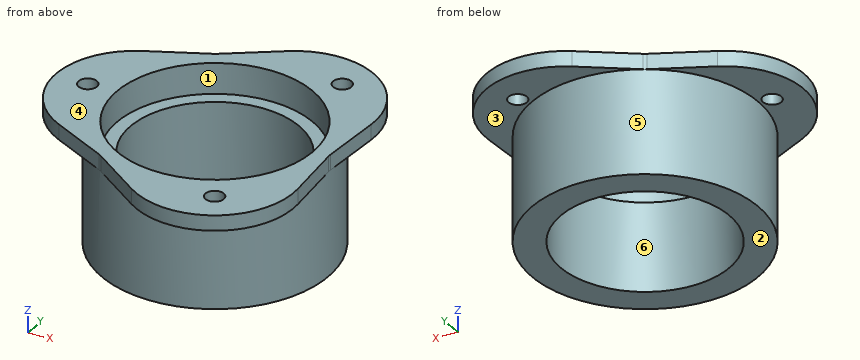
Autodesk Inventor part; units mm, degrees
ref_plane "XZ Plane" through (0, 0, 0) normal (0, 1, 0) x (-1, 0, 0)
ref_plane "XY Plane" through (0, 0, 0) normal (0, 0, 1) x (1, 0, 0)
sketch "Sketch1" plane through (0, 0, 0) normal (0, 0, 1) x (1, 0, 0)
  circle A0 centre (0, 0) radius 27.575
  circle A1 centre (0, 0) radius 51.5
  dimension "d0" = 55.15
  dimension "d1" = 103
extrude "Extrusion1" add sketch "Sketch1" along normal blind 39
sketch "Sketch2" plane through (0, 0, 0) normal (1, 0, 0) x (0, 1, 0)
  line L0 (51.5, 39) -> (-51.5, 39)
  line L1 (51.5, 0) -> (-51.5, 0)
  line L2 (42.7787, 29) -> (-54.5799, 29) construction
  line L3 (-27.575, 39) -> (27.575, 39)
  line L4 (-27.575, 39) -> (27.575, 39)
  line L5 (-27.575, 0) -> (27.575, 0)
  line L6 (51.5, 0) -> (27.575, 0)
  line L7 (27.575, 0) -> (27.575, 39)
  line L8 (27.575, 39) -> (51.5, 39)
  line L9 (-51.5, 39) -> (-27.575, 39)
  line L10 (-27.575, 39) -> (-27.575, 0)
  line L11 (-27.575, 0) -> (-51.5, 0)
  line L12 (27.575, 39) -> (32, 39)
  line L13 (32, 39) -> (32, 29)
  line L14 (32, 29) -> (27.575, 29)
  line L15 (27.575, 29) -> (27.575, 39)
  line L16 (0, -7.8) -> (0, 46.8)
  line L17 (51.5, 39) -> (51.5, 0)
  line L18 (-51.5, 0) -> (-51.5, 39)
  point P0 (0, 0)
  dimension "d4" = 10
  dimension "d5" = 32
revolve "Revolution1" cut sketch "Sketch2" angle 360 about axis through (0, 0, -10) along (0, 0, 1) contours L13 L14 L7 L0
sketch "Sketch3" plane through (0, 0, 0) normal (1, 0, 0) x (0, 1, 0)
  line L0 (51.5, 39) -> (51.5, 0)
  line L1 (51.5, 0) -> (27.575, 0)
  line L2 (27.575, 0) -> (27.575, 29)
  line L3 (27.575, 29) -> (32, 29)
  line L4 (32, 29) -> (32, 39)
  line L5 (32, 39) -> (51.5, 39)
  line L6 (-51.5, 0) -> (-51.5, 39)
  line L7 (-51.5, 39) -> (-32, 39)
  line L8 (-32, 39) -> (-32, 29)
  line L9 (-32, 29) -> (-27.575, 29)
  line L10 (-27.575, 29) -> (-27.575, 0)
  line L11 (-27.575, 0) -> (-51.5, 0)
  line L12 (-51.5, 0) -> (-51.5, 39)
  line L13 (-32, 39) -> (-32, 29)
  line L14 (-32, 34) -> (-51.5, 34)
  line L15 (-37, 34) -> (-37, 0)
  line L16 (51.5, 0) -> (-51.5, 0)
  line L17 (0, -7.8) -> (0, 46.8)
  point P0 (0, 0)
  point P1 (-51.5, 34)
  dimension "d7" = 5
  dimension "d11" = 5
revolve "Revolution2" cut sketch "Sketch3" angle 360 about axis through (0, 0, -10) along (0, 0, 1) contours L11 L6 L14 L15
sketch "Sketch4" plane through (0, 0, 39) normal (0, 0, 1) x (1, 0, 0)
  circle A0 centre (0, 0) radius 32
  circle A1 centre (0, 0) radius 51.5
  circle A2 centre (0, 0) radius 32
  line L0 (0, 0) -> (-55.0177, 0) construction
  line L1 (0, 0) -> (34.9883, -60.6016) construction
  line L2 (0, 0) -> (42.9469, 74.3862) construction
  circle A3 centre (-25.75, 0) radius 25.75 construction
  circle A4 centre (12.875, -22.3002) radius 25.75 construction
  circle A5 centre (0, 0) radius 51.5
  circle A6 centre (12.875, 22.3002) radius 25.75 construction
  line L3 (0, 0) -> (-33.8932, -58.7048) construction
  line L4 (0, 0) -> (-35.029, 60.6721) construction
  line L5 (0, 0) -> (41.9391, 0) construction
  circle A7 centre (-22.125, -38.3216) radius 7.25 construction
  circle A8 centre (-22.125, 38.3216) radius 7.25 construction
  circle A9 centre (44.25, 0) radius 7.25 construction
  line L6 (38.5484, -20.3161) -> (37.0216, -0.5586)
  line L7 (38.5484, 20.3161) -> (37.0216, 0.5586)
  line L8 (-1.68, -43.542) -> (-18.027, -32.3409)
  line L9 (-36.8684, -23.2259) -> (-18.9946, -31.7823)
  line L10 (-36.8684, 23.2259) -> (-18.9946, 31.7823)
  line L11 (-18.027, 32.3409) -> (-1.68, 43.542)
  arc A10 (-1.68, -43.542) -> (38.5484, -20.3161) centre (12.875, -22.3002) ccw
  arc A11 (37.0216, 0.5586) -> (37.0216, -0.5586) centre (44.25, 0) ccw
  arc A12 (36.3356, 11.6859) -> (-1.68, 43.542) centre (12.875, 22.3002) ccw
  arc A13 (-18.9946, 31.7823) -> (-18.027, 32.3409) centre (-22.125, 38.3216) ccw
  arc A14 (-18.027, -32.3409) -> (-18.9946, -31.7823) centre (-22.125, -38.3216) ccw
  arc A15 (-36.8684, 23.2259) -> (-36.8684, -23.2259) centre (-25.75, 0) ccw
  circle A16 centre (0, 0) radius 37
  point P0 (-51.5, 0)
  point P1 (25.75, -44.6003)
  point P2 (25.75, 44.6003)
  dimension "d12" = 120
  dimension "d13" = 120
  dimension "d14" = 120
  dimension "d15" = 120
extrude "Extrusion2" cut sketch "Sketch4" against normal up to surface (5 mm away) contours A1 A10 L6 A11 L7 A12 | A12 L11 A13 L10 A15 A1 | A1 A15 L9 A14 L8 A10
sketch "Sketch5" plane through (0, 0, 39) normal (0, 0, 1) x (1, 0, 0)
  circle A0 centre (0, 0) radius 32
  line L0 (0, 0) -> (-33.178, 0) construction
  circle A1 centre (-41, 0) radius 3
  point P0 (20.5, -35.507)
  point P1 (20.5, 35.507)
  dimension "d18" = 6
  dimension "d19" = 41
  dimension "d22" = 360
hole "Hole1" at (-41, 0, 39) at (20.5, 35.507, 39) at (20.5, -35.507, 39) direction (0, 0, -1) diameter 6 end through all
equation "\"d13\" = d12"
equation "\"d14\" = d12"
equation "\"d15\" = d12"
properties part number "EDF Mount"
For this review, take the finished solid that the model builds, in its own axes (mm). Face numbers are marked on the shaded views. A direction names the side the tool comes from. Round coordinates to 2 decimals unless told otherwise and drop trailing zeros. Write each loop counter-clockwise with the first axis right and the second up, starting at its lowest first coordinate (ties: lowest second). Pieces come first, ordered by that corner, then holes. Notation, with made-up numbers: (-12, 63.5) - (28, 63.5) arc R6 ccw to (28, 69.5) - close; hole circle Ø10 at (65.5, -7). An arc over 180 degrees is marked (long way). Answer as a JSON object with one key per item and string values.
1. Tool access review of the marked faces 1, 2 and 3: name each direction out of +Z, -Z, +X, -X, +Y, -Y from which nothing blocks a thin tool from reaching the whole face with its end or side.
Response values:
{"face 1": "+Z", "face 2": "-Z, +X, -X, +Y, -Y", "face 3": "-Z"}
2. Draft analysis for pull direction Y (two halves, no side actions). For the marked faces 4, 5 and 6, state which applies: +Y half, -Y half, draft (parallel to the pull), parting line (faces both ways), or undercut.
Response values:
{"face 4": "draft", "face 5": "parting line", "face 6": "undercut"}
3. We need section D-D on z = 27. Give the boundary of the cut face in (x, y) (3 decimals).
Response values:
{"outline": "circle Ø74 at (0, 0); hole circle Ø55.15 at (0, 0)"}
4. We need section A-A on x = -23. Give the boundary of the cut face in (y, z), then the cut area to 3 significant figures.
Response values:
{"outline": "(-29.86, 34) - (-28.98, 34) - (-28.98, 0) - (-15.21, 0) - (-15.21, 29) - (-22.25, 29) - (-22.25, 39) - (-29.86, 39) - close; (15.21, 0) - (28.98, 0) - (28.98, 34) - (29.86, 34) - (29.86, 39) - (22.25, 39) - (22.25, 29) - (15.21, 29) - close", "area": "942 mm2"}
5. To check wall thickness, follow line 1 along X through (y, z) = (0, 37.25); line 2 along Y through (x, z) = (20.5, 37.45); line 3 along Y through (x, z) = (0, 33). State the ranges of each line that lie inside material, in increasing order.
Response values:
{"line 1": "x = -51.5 to -44, -38 to -32, 32 to 37", "line 2": "y = -46.9 to -38.51, -32.51 to -24.57, 24.57 to 32.51, 38.51 to 46.9", "line 3": "y = -37 to -32, 32 to 37"}
6. We need section C-C on x = 20.5. Give the boundary of the cut face in (y, z).
Response values:
{"outline": "(-46.9, 34) - (-38.51, 34) - (-38.51, 39) - (-46.9, 39) - close; (-32.51, 34) - (-30.8, 34) - (-30.8, 0) - (-18.44, 0) - (-18.44, 29) - (-24.57, 29) - (-24.57, 39) - (-32.51, 39) - close; (18.44, 0) - (30.8, 0) - (30.8, 34) - (32.51, 34) - (32.51, 39) - (24.57, 39) - (24.57, 29) - (18.44, 29) - close; (38.51, 34) - (46.9, 34) - (46.9, 39) - (38.51, 39) - close"}
7. For pin 1 Ø6 at (x, z) = (25.5, 8.5) entering from +Y; pin 2 Ø8 at (y, z) = (15, 30.5) entering from +X; pin 3 Ø3 at (x, z) = (-22.5, 29) entering from -Y, all flat-tipped, find the tip position at first contact; note any pin that passes through.
Response values:
{"pin 1": "stops at y = 29.37", "pin 2": "stops at x = 38.29", "pin 3": "stops at y = -30.46"}
8. We need section B-B on y = -9.5. Give the boundary of the cut face in (x, z).
Response values:
{"outline": "(-49.68, 34) - (-35.76, 34) - (-35.76, 0) - (-25.89, 0) - (-25.89, 29) - (-30.56, 29) - (-30.56, 39) - (-49.68, 39) - close; (25.89, 0) - (35.76, 0) - (35.76, 34) - (37.71, 34) - (37.71, 39) - (30.56, 39) - (30.56, 29) - (25.89, 29) - close"}
